CAD build for the part. Positions are in the model's coordinates, mm. A direction names the side the tool comes from. Give positions to 0.01 mm unless a question says otherwise; leave off trailing zeros. Order: outer loops, then holes, each group sorted by start corner. A loop starts at its lowest first (then second) coordinate and runs counter-clockwise, first axis right, second up.
```python
from build123d import *

# Parameters (mm, degrees)
SKETCH_1_W             = 37.9
SKETCH_1_H             = 17.9
EXTRUDE_1_DEPTH        = 20
CHAMFER_1_SIZE         = 0.8
FILLET_1_R             = 0.5
SKETCH_2_R             = 6.5
CUT_EXTRUDE_1_DEPTH    = 4.05
SKETCH_3_R             = 5
CUT_EXTRUDE_2_DEPTH    = 64
CHAMFER_2_SIZE         = 0.3
HOLE_WIZARD_M4_1_D     = 3.3
HOLE_WIZARD_M4_1_DEPTH = 20
HOLE_WIZARD_M4_1_TIP   = 0.991420021
HOLE_WIZARD_M4_2_D     = 3.3
HOLE_WIZARD_M4_2_DEPTH = 42.1
HOLE_WIZARD_M4_2_TIP   = 0.991420021
EXTRUDE_2_DEPTH        = 10
SKETCH_17_W            = 20.1
SKETCH_17_H            = 46
CUT_EXTRUDE_5_DEPTH    = 25
FILLET_2_R             = 2
SKETCH_18_R            = 2.1
CUT_EXTRUDE_6_DEPTH    = 35
FILLET_4_R             = 2
HOLE_WIZARD_M4_4_D     = 3.3
HOLE_WIZARD_M4_4_DEPTH = 42.1
HOLE_WIZARD_M4_4_TIP   = 0.991420021


# Some blends are built 0.0001 mm under size
with BuildPart() as part:
    # 草图1 → 凸台-拉伸1 (new, symmetric)
    with BuildSketch(Plane.XY):
        Rectangle(SKETCH_1_W, SKETCH_1_H)
    extrude(amount=EXTRUDE_1_DEPTH, both=True)

    # 倒角1
    chamfer_1_edges = [part.edges().sort_by_distance(p)[0] for p in [
        (-18.95, -8.95, 0),
        (-18.95, 8.95, 0),
        (18.95, 8.95, 0),
        (18.95, -8.95, 0),
    ]]
    chamfer(chamfer_1_edges, length=CHAMFER_1_SIZE)

    # 圆角1
    fillet_1_edges = [part.edges().sort_by_distance(p)[0] for p in [
        (18.15, -8.95, 0),
        (-18.15, -8.95, 0),
        (-18.95, 8.15, 0),
        (-18.95, -8.15, 0),
        (18.95, 8.15, 0),
        (18.95, -8.15, 0),
        (18.15, 8.95, 0),
        (-18.15, 8.95, 0),
    ]]
    fillet(fillet_1_edges, radius=FILLET_1_R)

    # 草图2 → 切除-拉伸1 (cut)
    with BuildSketch(Plane.ZY.offset(18.95)):
        with Locations((-9, 0)):
            Circle(SKETCH_2_R)
    cut_extrude_1 = extrude(amount=-CUT_EXTRUDE_1_DEPTH, mode=Mode.SUBTRACT)

    # 草图3 → 切除-拉伸2 (cut)
    with BuildSketch(Plane.ZY.offset(14.9)):
        with Locations((-9, 0)):
            Circle(SKETCH_3_R)
    extrude(amount=-CUT_EXTRUDE_2_DEPTH, mode=Mode.SUBTRACT)

    # 镜向1: 切除-拉伸1 across plane
    add(cut_extrude_1.mirror(Plane(origin=(0, 0, 0), x_dir=(0, 0, 1), z_dir=(1, 0, 0))), mode=Mode.SUBTRACT)

    # 倒角2
    chamfer_2_edges = [part.edges().sort_by_distance(p)[0] for p in [
        (-18.95, 0, -15.5),
        (18.95, 0, -15.5),
    ]]
    chamfer(chamfer_2_edges, length=CHAMFER_2_SIZE)

    # M4 螺纹孔1
    with Locations(Plane(origin=(0, 8.95, 0), x_dir=(1, 0, 0), z_dir=(0, 1, 0))):
        with Locations((-14.5, -0.5), (14.5, -0.5)):
            Hole(HOLE_WIZARD_M4_1_D / 2, depth=HOLE_WIZARD_M4_1_DEPTH)
            with Locations((0, 0, -(HOLE_WIZARD_M4_1_DEPTH + HOLE_WIZARD_M4_1_TIP / 2))):  # 118° drill point
                Cone(0, HOLE_WIZARD_M4_1_D / 2, HOLE_WIZARD_M4_1_TIP, mode=Mode.SUBTRACT)

    # M4 螺纹孔2
    with Locations(Plane(origin=(18.95, 0, 0), x_dir=(0, 0, -1), z_dir=(1, 0, 0))):
        with Locations((-9, 5), (-9, -5)):
            Hole(HOLE_WIZARD_M4_2_D / 2, depth=HOLE_WIZARD_M4_2_DEPTH)
            with Locations((0, 0, -(HOLE_WIZARD_M4_2_DEPTH + HOLE_WIZARD_M4_2_TIP / 2))):  # 118° drill point
                Cone(0, HOLE_WIZARD_M4_2_D / 2, HOLE_WIZARD_M4_2_TIP, mode=Mode.SUBTRACT)

    # 草图13 → 凸台-拉伸2 (add)
    with BuildSketch(Plane.XY.offset(20)):
        with BuildLine():
            Line((-17.942893219, -8.95), (17.942893219, -8.95))
            ThreePointArc((17.942893219, -8.95), (18.134234935, -8.911939766), (18.296446609, -8.803553391))
            Line((18.296446609, -8.803553391), (18.803553391, -8.296446609))
            ThreePointArc((18.803553391, -8.296446609), (18.911939766, -8.134234935), (18.95, -7.942893219))
            Line((18.95, -7.942893219), (18.95, 7.942893219))
            ThreePointArc((18.95, 7.942893219), (18.911939766, 8.134234935), (18.803553391, 8.296446609))
            Line((18.803553391, 8.296446609), (18.296446609, 8.803553391))
            ThreePointArc((18.296446609, 8.803553391), (18.134234935, 8.911939766), (17.942893219, 8.95))
            Line((17.942893219, 8.95), (-17.942893219, 8.95))
            ThreePointArc((-17.942893219, 8.95), (-18.134234935, 8.911939766), (-18.296446609, 8.803553391))
            Line((-18.296446609, 8.803553391), (-18.803553391, 8.296446609))
            ThreePointArc((-18.803553391, 8.296446609), (-18.911939766, 8.134234935), (-18.95, 7.942893219))
            Line((-18.95, 7.942893219), (-18.95, -7.942893219))
            ThreePointArc((-18.95, -7.942893219), (-18.911939766, -8.134234935), (-18.803553391, -8.296446609))
            Line((-18.803553391, -8.296446609), (-18.296446609, -8.803553391))
            ThreePointArc((-18.296446609, -8.803553391), (-18.134234935, -8.911939766), (-17.942893219, -8.95))
        make_face()
    extrude(amount=EXTRUDE_2_DEPTH)

    # 草图17 → 切除-拉伸5 (cut)
    with BuildSketch(Plane(origin=(0, 8.95, 0), x_dir=(1, 0, 0), z_dir=(0, 1, 0))):
        with Locations((0, -7)):
            Rectangle(SKETCH_17_W, SKETCH_17_H)
    extrude(amount=-CUT_EXTRUDE_5_DEPTH, mode=Mode.SUBTRACT)

    # 圆角2
    fillet_2_edges = [part.edges().sort_by_distance(p)[0] for p in [
        (-10.05, 0, -16),
        (10.05, 0, -16),
    ]]
    fillet(fillet_2_edges, radius=FILLET_2_R - 0.0001)  # a hair under: the kernel refuses the full size
    fillet_2_2_edges = [part.edges().sort_by_distance(p)[0] for p in [
        (10.05, 0, 30),
        (-10.05, 0, 30),
    ]]
    fillet(fillet_2_2_edges, radius=FILLET_2_R)

    # 草图18 → 切除-拉伸6 (cut)
    with BuildSketch(Plane.XZ.offset(8.95)):
        with Locations(Location((-14.5, 19, 0), (0, 0, 270))):
            Circle(SKETCH_18_R)
        with Locations(Location((14.5, 19, 0), (0, 0, 270))):
            Circle(SKETCH_18_R)
    extrude(amount=-CUT_EXTRUDE_6_DEPTH, mode=Mode.SUBTRACT)

    # 圆角4
    # the kernel refuses this fillet: 2 mm, written as the material it takes off along each edge
    with BuildSketch(Plane(origin=(-18.95, -12.942893219, -20), x_dir=(1, 0, 0), z_dir=(0, 1, 0)), Plane(origin=(18.95, 12.942893219, -20), x_dir=(-1, 0, 0), z_dir=(0, -1, 0)), Plane(origin=(18.95, -12.942893219, 30), x_dir=(-1, 0, 0), z_dir=(0, 1, 0)), Plane(origin=(-18.95, 12.942893219, 30), x_dir=(1, 0, 0), z_dir=(0, -1, 0))) as fillet_4_piece_1:
        with BuildLine():
            CenterArc((FILLET_4_R, -FILLET_4_R), FILLET_4_R, 90, 90)
            Line((0, -FILLET_4_R), (0, 0))
            Line((0, 0), (FILLET_4_R, 0))
        make_face()
    extrude(amount=25.885786438, mode=Mode.SUBTRACT)

    # M4 螺纹孔4
    with Locations(Plane(origin=(18.95, 0, 0), x_dir=(0, 0, -1), z_dir=(1, 0, 0))):
        with Locations((-24, 5), (-24, -5)):
            Hole(HOLE_WIZARD_M4_4_D / 2, depth=HOLE_WIZARD_M4_4_DEPTH)
            with Locations((0, 0, -(HOLE_WIZARD_M4_4_DEPTH + HOLE_WIZARD_M4_4_TIP / 2))):  # 118° drill point
                Cone(0, HOLE_WIZARD_M4_4_D / 2, HOLE_WIZARD_M4_4_TIP, mode=Mode.SUBTRACT)


solid = part.part
```
Item 1: Slice it at C-C (z = 19). Give the cut face in (x, y), and give its area (3 significant figures).
Item 2: Slice it at D-D (x = 2). Give the cut face in (y, z).
Item 3: Wall check: L1, parallel to X at y = -3, z = 12.5; L2, parallel to Y at x = 12, z = -9. Give the ranges that are in metal, low to high.
Item 4: Drop a flat-ended pin along its axis: pin 1 Ø6.5 at (y, z) = (0.5, -6.5) entering from +X. Give the stop position or say it passes through.
Item 5: Tool access for faces 5 (the face through (10.05, 0, 7)), 6 (the face through (16.8, 1.95, -2.8)), 7 (the face through (12, -8.95, 5)): list every direction of +Z, -Z, +X, -X, +Y, -Y with a clear straight run to the whole face (end or side of a thin tool).
Item 6: Slice it at A-A (z = 0.5). Give the cut face in (x, y).
Item 7: Two-plate mould, pull along X, no slides. Class faces 1 (the face through (-9.45, -0.13, -15.43)), 2 (the face through (14.9, -5, -7)), 3 (the face through (10.62, -0.13, 29.4)), 4 (the face through (14.44, -6, 7.69)): released by +X, released by -X, zero draft, split by the parting line, or undercut.
Item 8: Slice it at B-B (y = 0). State how many separate pieces and enclosed holes the cut face has, and give its area (3 significant figures).
A:
1. outline: (-18.95, -7.94) arc R0.5 ccw to (-18.8, -8.3) - (-18.3, -8.8) arc R0.5 ccw to (-17.94, -8.95) - (-16.6, -8.95) - (-16.6, 8.95) - (-17.94, 8.95) arc R0.5 ccw to (-18.3, 8.8) - (-18.8, 8.3) arc R0.5 ccw to (-18.95, 7.94) - close; (-12.4, -8.95) - (-10.05, -8.95) - (-10.05, 8.95) - (-12.4, 8.95) - close; (10.05, -8.95) - (12.4, -8.95) - (12.4, 8.95) - (10.05, 8.95) - close; (16.6, -8.95) - (17.94, -8.95) arc R0.5 ccw to (18.3, -8.8) - (18.8, -8.3) arc R0.5 ccw to (18.95, -7.94) - (18.95, 7.94) arc R0.5 ccw to (18.8, 8.3) - (18.3, 8.8) arc R0.5 ccw to (17.94, 8.95) - (16.6, 8.95) - close
1. area: 167 mm2
2. outline: (-8.95, -20) - (8.95, -20) - (8.95, -16) - (-8.95, -16) - close
3. L1: x = -18.95 to -10.05, 10.05 to 18.95
3. L2: y = -8.95 to -5, 5 to 8.95
4. pin 1: stops at x = 14.9
5. face 5: +Z, +Y, -Y
5. face 6: +X
5. face 7: +Z, -Z, +X, -X, -Y
6. outline: (-18.95, -7.94) arc R0.5 ccw to (-18.8, -8.3) - (-18.3, -8.8) arc R0.5 ccw to (-17.94, -8.95) - (-16.15, -8.95) - (-16.15, 8.95) - (-17.94, 8.95) arc R0.5 ccw to (-18.3, 8.8) - (-18.8, 8.3) arc R0.5 ccw to (-18.95, 7.94) - close; (-12.85, -8.95) - (-10.05, -8.95) - (-10.05, 8.95) - (-12.85, 8.95) - close; (10.05, -8.95) - (12.85, -8.95) - (12.85, 8.95) - (10.05, 8.95) - close; (16.15, -8.95) - (17.94, -8.95) arc R0.5 ccw to (18.3, -8.8) - (18.8, -8.3) arc R0.5 ccw to (18.95, -7.94) - (18.95, 7.94) arc R0.5 ccw to (18.8, 8.3) - (18.3, 8.8) arc R0.5 ccw to (17.94, 8.95) - (16.15, 8.95) - close
7. face 1: undercut
7. face 2: released by +X
7. face 3: undercut
7. face 4: zero draft
8. separate pieces: 3
8. enclosed holes: 4
8. area: 720 mm2
